```python
from build123d import *

# Parameters (mm, degrees)
EXTRUDE_1_DEPTH     = 87.5
CUT_EXTRUDE_1_DEPTH = 175
SKETCH_3_R          = 12
CUT_EXTRUDE_2_DEPTH = 52
SKETCH_4_R          = 5.5
CUT_EXTRUDE_3_DEPTH = 40
FILLET_1_R          = 5


with BuildPart() as part:
    # 草图1 → 凸台-拉伸1 (new, symmetric)
    with BuildSketch(Plane.XY):
        Polygon((0, 0), (0, 60), (75, 50), (75, 0), align=None)
    extrude(amount=EXTRUDE_1_DEPTH, both=True)

    # 草图2 → 切除-拉伸1 (cut)
    with BuildSketch(Plane.XZ):
        Polygon((0, 87.5), (75, 67.5), (75, 87.5), align=None)
        Polygon((0, -87.5), (75, -67.5), (75, -87.5), align=None)
    extrude(amount=-CUT_EXTRUDE_1_DEPTH, mode=Mode.SUBTRACT)

    # 草图3 → 切除-拉伸2 (cut)
    with BuildSketch(Plane(origin=(75, 0, 0), x_dir=(0, 0, -1), z_dir=(1, 0, 0))):
        with Locations((-27.5, 25)):
            Circle(SKETCH_3_R)
        with Locations((27.5, 25)):
            Circle(SKETCH_3_R)
    extrude(amount=-CUT_EXTRUDE_2_DEPTH, mode=Mode.SUBTRACT)

    # 草图4 → 切除-拉伸3 (cut)
    with BuildSketch(Plane(origin=(23, 0, 0), x_dir=(0, 0, -1), z_dir=(1, 0, 0))):
        with Locations((-27.5, 25)):
            Circle(SKETCH_4_R)
        with Locations((27.5, 25)):
            Circle(SKETCH_4_R)
    extrude(amount=-CUT_EXTRUDE_3_DEPTH, mode=Mode.SUBTRACT)

    # 圆角1
    fillet_1_edges = [part.edges().sort_by_distance(p)[0] for p in [
        (75, 50, 0),
        (75, 0, 0),
        (37.5, 55, 77.5),
        (75, 25, 67.5),
        (37.5, 0, 77.5),
        (75, 25, -67.5),
        (37.5, 55, -77.5),
        (37.5, 0, -77.5),
    ]]
    fillet(fillet_1_edges, radius=FILLET_1_R)


solid = part.part
```
Build history of the part. All positions in model axes, mm. A direction names the side the tool comes from. Coordinates: 2 decimals unless noted, no trailing zeros. Order: outer loops, then holes, each group sorted by start corner. A loop starts at its lowest first (then second) coordinate and runs counter-clockwise, first axis right, second up. Notation, with made-up numbers: M 66,-37.75 L 85,-37.75 A18 cw 85,-2.75 Z; hole C 8.5,12 d2. An arc over 180 degrees is marked long. One line per question, with ' | ' between items. Start each with the question number.
1. Flat gauge pins, fed straight in: P1, Ø7, axis at y = 24.5, z = 30, coming from the +X side; P2, Ø4, axis at x = 25.5, z = 33, coming from the +Y side; P3, Ø4, axis at x = 24.5, z = 21, coming from the +Y side. Where does each tip first touch, or does it go through?
2. Cut at A-A (y = 25). Write the cut outline in (x, z), plus the area to 3 significant figures.
3. Tool access for faces 1 (the face through (49.364, 20.404, -38.585)), 2 (the face through (12, 25, -22)): list every direction of +Z, -Z, +X, -X, +Y, -Y with a clear straight run to the whole face (end or side of a thin tool).
4. Cut at B-B (z = 27.5). Write the cut outline in (x, y), plus the area to 3 significant figures.
5. Cut at C-C (z = 1). Write the cut outline in (x, y), plus the area to 3 significant figures.
6. Cut at D-D (y = 11). Write the cut outline in (x, z).
7. Wall check: line 1 along Z through (x, y) = (42, 26); line 2 along X through (y, z) = (33, -24.5); line 3 along Y through (x, z) = (6, -27.5). Give the ranges that are in metal, low to high. Write a range as [from, to].
8. Mould opens along Y. For faces 3 (the face through (23, 23, -33)), 4 (the face through (36.1, 53.73, -76.46)), 5 (the face through (73.94, 25.6, 66.74)) say: +Y half, -Y half, draft (parallel to the pull), parting line (faces both ways), or undercut.
The answers:
1) P1: stops at x = 23 | P2: stops at y = 56.87 | P3: stops at y = 57
2) outline: M 0,-87.5 L 71.29,-68.49 A5 ccw 75,-63.66 L 75,-39.5 L 23,-39.5 L 23,-33 L 0,-33 Z; M 0,-22 L 23,-22 L 23,-15.5 L 75,-15.5 L 75,15.5 L 23,15.5 L 23,22 L 0,22 Z; M 0,33 L 23,33 L 23,39.5 L 75,39.5 L 75,63.66 A5 ccw 71.29,68.49 L 0,87.5 Z | area: 8,620 mm2
3) face 1: +X | face 2: +X, -X
4) outline: M 0,0 L 70,0 A5 ccw 75,5 L 75,13 L 23,13 L 23,19.5 L 0,19.5 Z; M 0,30.5 L 23,30.5 L 23,37 L 75,37 L 75,45.62 A5 ccw 70.66,50.58 L 0,60 Z | area: 2,610 mm2
5) outline: M 0,0 L 70,0 A5 ccw 75,5 L 75,45.62 A5 ccw 70.66,50.58 L 0,60 Z | area: 4,120 mm2
6) outline: M 0,-87.5 L 71.29,-68.49 A5 ccw 75,-63.66 L 75,63.66 A5 ccw 71.29,68.49 L 0,87.5 Z
7) line 1: z = [-76.3, -39.46], [-15.54, 15.54], [39.46, 76.3] | line 2: x = [0, 23] | line 3: y = [0, 19.5], [30.5, 59.2]
8) face 3: undercut | face 4: +Y half | face 5: draft
